Source: three-view drawing plus pictorial views. Frame: mm from the lowest corner of the part. A direction names the side the tool comes from. Give positions to 0.01 mm unless a question says otherwise; leave off trailing zeros. Write each loop counter-clockwise with the first axis right and the second up, starting at its lowest first coordinate (ties: lowest second). Pieces come first, ordered by that corner, then holes. Notation, with made-up numbers: (79.25, 31) -> (123.25, 31) arc R27 cw to (123.25, 66) -> close; hole circle Ø1 at (8, 58.5). An arc over 180 degrees is marked (long way). Write item = value, one per line.
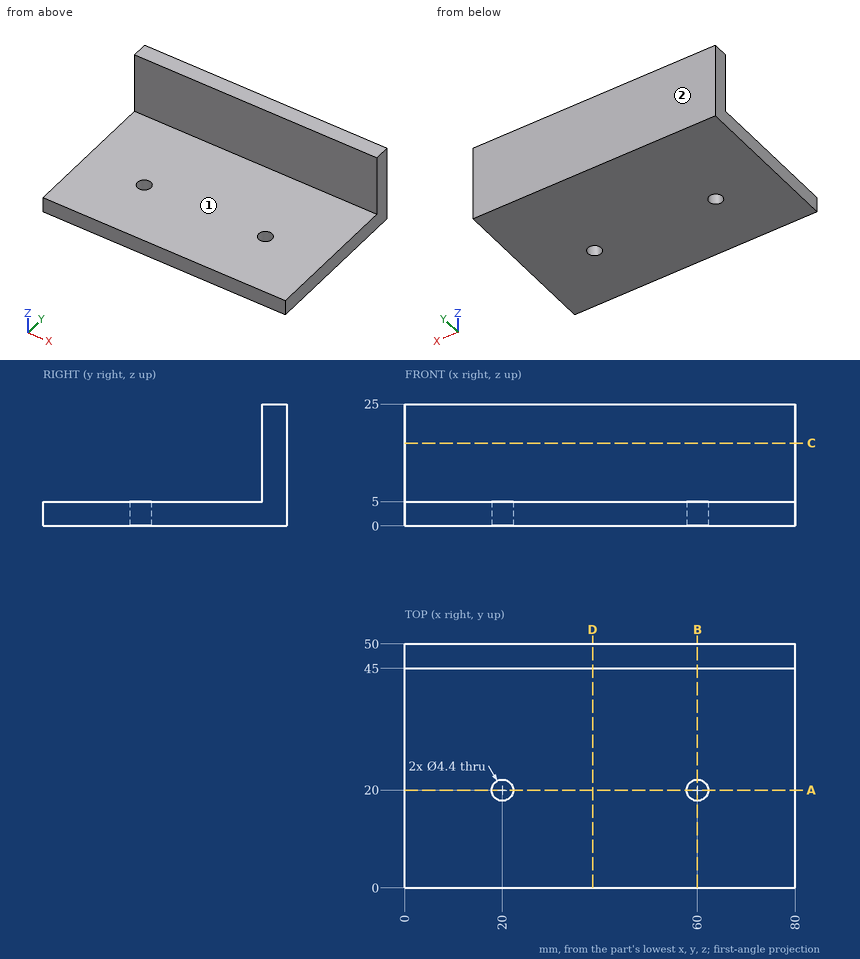
1) Access query for the marked faces 1 and 2. Directions: +Z, -Z, +X, -X, +Y, -Y. A direction counts if a zero-diameter tool reaches every point of the face in a straight line with its end or side. Return the directions, or none.
Computed:
face_1 = +Z, +X, -X, -Y
face_2 = +Z, -Z, +X, -X, +Y
2) Contact query for flat-ended pins moving along their axis: pin 1 (10 mm diameter, centred on x = 52, z = 13.5, fed in from -Y); pin 2 (1 mm diameter, centred on x = 51.5, y = 43.5, fed in from +Z); pin 3 (5 mm diameter, centred on y = 40, z = 8.5, fed in from +X). Output: stop coordinate, or through.
Computed:
pin_1 = 45
pin_2 = 5
pin_3 = through
3) Cut plane C-C (z = 17). Return the cut outline in (x, y), then the cut area to 3 significant figures.
Computed:
outline = (0, 45) -> (80, 45) -> (80, 50) -> (0, 50) -> close
area = 400 mm²
4) Cut plane D-D (x = 38.5). Return the cut outline in (y, z).
Computed:
outline = (0, 0) -> (50, 0) -> (50, 25) -> (45, 25) -> (45, 5) -> (0, 5) -> close
5) Cut plane B-B (x = 60). Return the cut outline in (y, z), then the cut area to 3 significant figures.
Computed:
outline = (0, 0) -> (17.8, 0) -> (17.8, 5) -> (0, 5) -> close; (22.2, 0) -> (50, 0) -> (50, 25) -> (45, 25) -> (45, 5) -> (22.2, 5) -> close
area = 328 mm²
6) Cut plane A-A (y = 20). Return the cut outline in (x, z), then the cut area to 3 significant figures.
Computed:
outline = (0, 0) -> (17.8, 0) -> (17.8, 5) -> (0, 5) -> close; (22.2, 0) -> (57.8, 0) -> (57.8, 5) -> (22.2, 5) -> close; (62.2, 0) -> (80, 0) -> (80, 5) -> (62.2, 5) -> close
area = 356 mm²
7) Material intervals for L1, parallel to Y at x = 20, z = 3.4; L2, parallel to Z at x = 55, y = 32; L3, parallel to Y at x = 47.5, z = 8.25, sorted ascending.
Computed:
L1 = 0 to 17.8, 22.2 to 50
L2 = 0 to 5
L3 = 45 to 50
